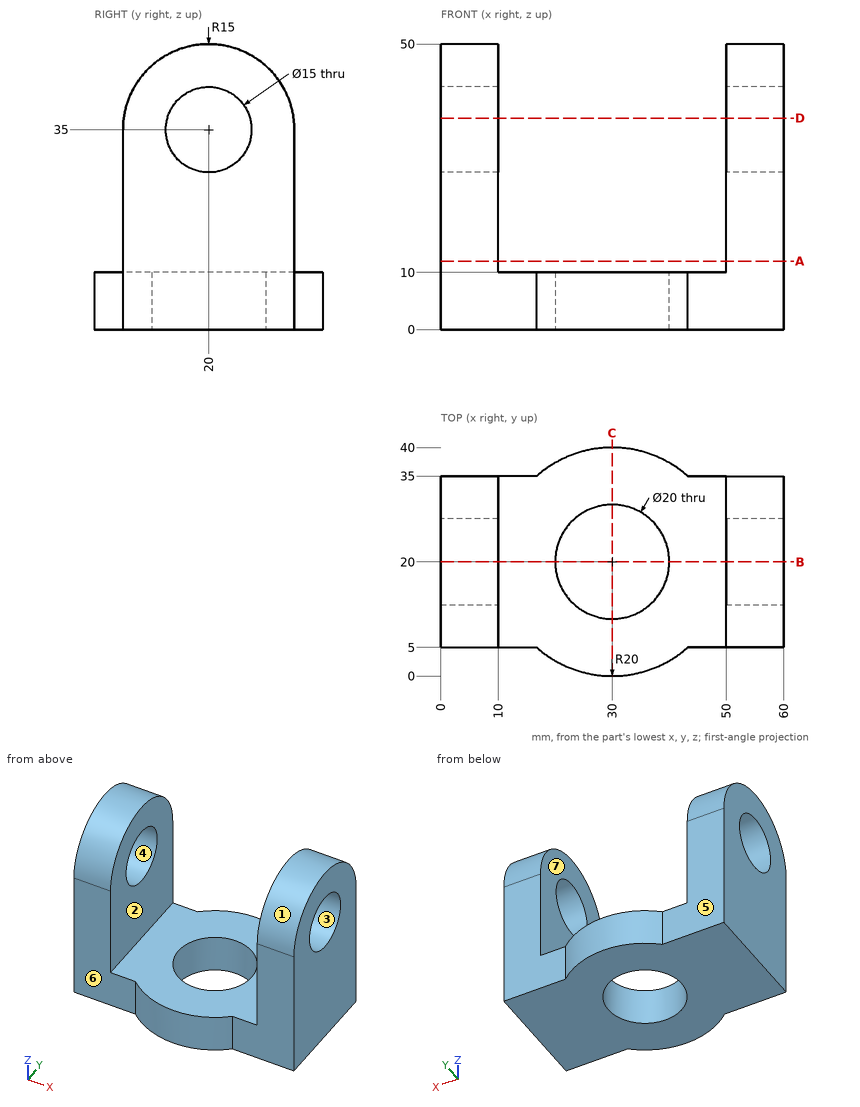
The drawing under review shows one solid part. Ordinate dimensions are in mm from its lowest x, y, z. A direction names the side the tool comes from. Give positions to 0.01 mm unless a question says otherwise; leave off trailing zeros. Loops run counter-clockwise (first coordinate to the right, second up) from the corner with the lowest first, then second, coordinate; pieces in that order, holes last. Notation, with made-up numbers: M -4,44 L 28,44 A22 cw 28,54 Z; hole C 83.5,-22 d11. An arc over 180 degrees is marked long. One line per question, with ' | ' between items. Start each with the question number.
1. For the marked faces 5, 6 and 7, list the 3-axis set-ups (+Z, -Z, +X, -X, +Y, -Y) from which the entire face can be reached by the end or side of a thin tool; tool diameter is ignored.
2. The part is to be moulded in two halves that separate along Z. For the marked faces 1, 2, 3 and 4, say which applies: released by +Z, released by -Z, zero draft, split by the parting line, or undercut.
3. To check wall thickness, follow L1, parallel to X at y = 23, z = 20; L2, parallel to Z at x = 54, y = 20; L3, parallel to Y at x = 37.5, z = 8.5. State the ranges of each line that lie inside material, in increasing order.
4. Add section A-A (z = 12). Write out the cut boundary in (x, y), plus the area to 3 significant figures.
5. Add section C-C (x = 30). Write out the cut boundary in (y, z).
6. Insertion check: P1, Ø20, axis at x = 21.5, y = 23, coming from the +Z side; P2, Ø8.5, axis at x = 10, z = 9, coming from the -Y side; P3, Ø13.5, axis at x = 5, z = 20.5, coming from the +Y side. Each pin has a flat end and moves straight along its axis. Give the tip position at first contact, or say it passes through.
7. Add section B-B (y = 20). Write out the cut boundary in (x, z), plus the area to 3 significant figures.
8. Add section D-D (z = 37). Write out the cut boundary in (x, y).
Worked out:
1) face 5: +Z, -Z, -X, +Y | face 6: +Z, -Z, -X, -Y | face 7: +Z, +Y, -Y
2) face 1: released by +Z | face 2: zero draft | face 3: undercut | face 4: undercut
3) L1: x = 0 to 10, 50 to 60 | L2: z = 0 to 27.5, 42.5 to 50 | L3: y = 1.46 to 13.39, 26.61 to 38.54
4) outline: M 0,5 L 10,5 L 10,35 L 0,35 Z; M 50,5 L 60,5 L 60,35 L 50,35 Z | area: 600 mm²
5) outline: M 0,0 L 10,0 L 10,10 L 0,10 Z; M 30,0 L 40,0 L 40,10 L 30,10 Z
6) P1: stops at z = 10 | P2: stops at y = 5 | P3: stops at y = 35
7) outline: M 0,0 L 20,0 L 20,10 L 10,10 L 10,27.5 L 0,27.5 Z; M 0,42.5 L 10,42.5 L 10,50 L 0,50 Z; M 40,0 L 60,0 L 60,27.5 L 50,27.5 L 50,10 L 40,10 Z; M 50,42.5 L 60,42.5 L 60,50 L 50,50 Z | area: 900 mm²
8) outline: M 0,5.13 L 10,5.13 L 10,12.77 L 0,12.77 Z; M 0,27.23 L 10,27.23 L 10,34.87 L 0,34.87 Z; M 50,5.13 L 60,5.13 L 60,12.77 L 50,12.77 Z; M 50,27.23 L 60,27.23 L 60,34.87 L 50,34.87 Z
